The listing builds one solid part. Answer for the finished solid, in the listing's coordinates (mm). A direction names the side the tool comes from. Give positions to 0.01 mm unless a question says otherwise; leave off trailing zeros. Write each loop counter-clockwise with the first axis right and the second up, starting at its lowest first coordinate (ties: lowest second). Pieces come first, ordered by that corner, then holes. Notation, with made-up numbers: M 46.5,83.25 L 104.5,83.25 A11 ccw 104.5,102.25 Z; hole C -17.75,47.5 d11. An arc over 180 degrees is marked long. Answer as a JSON object with one key per item and string values.
```python
from build123d import *

# Parameters (mm, degrees)
F0_R     = 30.1625
F0_R_2   = 15.875
F1_DEPTH = 41.275
F3_DEPTH = 15.875
F4_W     = 14.2875
F4_H     = 31.75
F5_DEPTH = 22.225
F7_DEPTH = 14.2875
F8_R     = 7.9375
F9_DEPTH = 25.4


with BuildPart() as f1:
    # F0 (on Front) → F1 (new body)
    with BuildSketch(Plane.XZ):
        with Locations((-43.274074, 0)):
            Circle(F0_R)
        with Locations((-43.274074, 0)):
            Circle(F0_R_2, mode=Mode.SUBTRACT)
    extrude(amount=F1_DEPTH)

    # F2 (on face) → F3 (join)
    with BuildSketch(Plane(origin=(0, 0, 0), x_dir=(-1, 0, 0), z_dir=(0, 1, 0))):
        with BuildLine():
            Line((-56.738426, -30.1625), (43.274074, -30.1625))
            ThreePointArc((43.274074, -30.1625), (13.429074, -4.364901), (34.636165, 28.899185))
            Line((34.636165, 28.899185), (-56.738426, 1.5875))
            Line((-56.738426, 1.5875), (-56.738426, -30.1625))
        make_face()
    extrude(amount=-F3_DEPTH)

    # F4 (on face) → F5 (join)
    with BuildSketch(Plane.XZ.offset(15.875)):
        with Locations((49.594676, -14.2875)):
            Rectangle(F4_W, F4_H)
    extrude(amount=F5_DEPTH)

    # F6 (on face) → F7 (join)
    with BuildSketch(Plane.YZ.offset(56.738426)):
        with BuildLine():
            Line((-38.1, -30.1625), (-38.1, 1.5875))
            ThreePointArc((-38.1, 1.5875), (-53.975, -14.2875), (-38.1, -30.1625))
        make_face()
    extrude(amount=-F7_DEPTH)

    # F8 (on face) → F9 (cut)
    with BuildSketch(Plane.YZ.offset(56.738426)):
        with Locations((-38.1, -14.2875)):
            Circle(F8_R)
    extrude(amount=-F9_DEPTH, mode=Mode.SUBTRACT)


solid = f1.part
```
1. A cutting plane is placed at A-A, the plane y = -27. Count the separate pieces of the cut face and the enclosed holes in it, plus the area to 3 significant figures.
Verdict:
{"separate pieces": "2", "enclosed holes": "1", "area": "2,520 mm2"}
2. A cutting plane is placed at B-B, the plane z = 8. Give the vertices of the cut face in (x, y) (3 decimals), plus the area to 3 significant figures.
Verdict:
{"outline": "M -72.356,-41.275 L -56.986,-41.275 L -56.986,0 L -72.356,0 Z; M -29.562,-41.275 L -14.192,-41.275 L -14.192,-15.875 L 35.285,-15.875 L 35.285,0 L -29.562,0 Z", "area": "2,050 mm2"}
3. A cutting plane is placed at D-D, the plane z = 0. Give the vertices of the cut face in (x, y) (3 decimals).
Verdict:
{"outline": "M -73.437,-41.275 L -59.149,-41.275 L -59.149,0 L -73.437,0 Z; M -27.399,-41.275 L -13.112,-41.275 L -13.112,-15.875 L 42.451,-15.875 L 42.451,-45.02 L 56.738,-45.02 L 56.738,0 L -27.399,0 Z"}
4. Consider line 1 along Y through (x, z) = (11, 4.5) (3 decimals); line 2 along Y through (x, z) = (-35, 21.5) (3 decimals); line 3 along Z through (x, y) = (-44, -4). Determine where each line is inside the solid, lowest interval first.
Verdict:
{"line 1": "y = -15.875 to 0", "line 2": "y = -41.275 to 0", "line 3": "z = -30.15 to -15.86, 15.86 to 30.15"}
5. Flat-ended cylindrical pins translate along their axes: pin 1 (1 mm diameter, centred on x = -53, y = -31.5, fed in from -Z); pin 2 (7 mm diameter, centred on x = 49.5, y = -27, fed in from +Z); pin 3 (17.5 mm diameter, centred on x = -9.5, z = 9.5, fed in from -Y) (3 decimals); pin 4 (10 mm diameter, centred on x = 37, y = -48.5, fed in from -Z). Find the tip coordinate at first contact, or state that the pin passes through.
Verdict:
{"pin 1": "stops at z = -28.72", "pin 2": "stops at z = 1.59", "pin 3": "stops at y = -41.275", "pin 4": "passes through"}
6. For faces 4 (the cylindrical face through (49.69, -53.97, -13.94)), 5 (the flat face through (49, -27, 1.588)), 6 (the cylindrical face through (49.69, -30.53, -11.9)), 7 (the flat face through (-30, -41.275, -13)), 8 (the cylindrical face through (-73.407, -24.935, 1.326)), determine the directions among +Z, -Z, +X, -X, +Y, -Y from which every point of the face is accessible in a straight line to the end or side of a thin tool.
Verdict:
{"face 4": "+X, -Y", "face 5": "+Z, +X, -Y", "face 6": "+X", "face 7": "+Z, -Z, -X, -Y", "face 8": "-Y"}
7. The mould has two halves that part along X. Classify faces 1 (the flat face through (56.738, -21, -14)), 2 (the flat face through (7, -15.875, -7)), 3 (the flat face through (-7, 0, -6)): released by +X, released by -X, zero draft, split by the parting line, or undercut.
Verdict:
{"face 1": "released by +X", "face 2": "undercut", "face 3": "zero draft"}
